The listing builds one solid part. Answer for the finished solid, in the listing's coordinates (mm). A direction names the side the tool comes from. Round coordinates to 2 decimals unless told otherwise and drop trailing zeros. Order: outer loops, then holes, each group sorted by start corner. A loop starts at its lowest first (then second) coordinate and runs counter-clockwise, first axis right, second up. Notation, with made-up numbers: (5, 33.5) -> (25, 33.5) arc R13 cw to (25, 45.5) -> close; hole circle Ø3 at (49, 71). An arc over 180 degrees is marked (long way). Return JSON: item names as keys, results as strings. Group by question number.
(1) Consider line 1 (Y direction, x = 0, z = 2.25); line 2 (Z direction, x = 4.25, y = -2); line 3 (Y direction, x = 0, z = 1.2). Determine where each line is inside the solid, lowest interval first. Write a range as [from, to].
(2) The part is cut by section A-A (z = 2.4). Count the separate pieces of the cut face and the enclosed holes in it, plus the area to 3 significant figures.
(3) The part is cut by section C-C (y = -4). Determine the outline of the cut face in (x, z).
(4) The part is cut by section D-D (y = 5.25). Determine the outline of the cut face in (x, z), plus the area to 3 significant figures.
(5) Each of these flat-tipped pins is pushed along its axis until it touches: pin 1 (4.5 mm diameter, centred on x = 0, y = 0, fed in from -Z); pin 2 (0.9 mm diameter, centred on x = -2, y = 4, fed in from +Z); pin 3 (0.5 mm diameter, centred on x = 1, y = 4, fed in from +Z). Where does it stop, or does it pass through?
(6) Determine the mould class of faces 3 (the face through (0.007, 4.1, 2.745)), 4 (the face through (1.2, -1.2, 1.6)), 5 (the face through (-1, 4, 2.1)), 6 (the face through (-2.894, 2.904, 2.745)) for opening direction X: +X half, -X half, draft (parallel to the pull), parting line (faces both ways), or undercut.
(7) Which of the six approach directions +Z, -Z, +X, -X, +Y, -Y give full straight-line access (tool end or side, diameter ignored) to faces 1 (the face through (4, 1, 2.1)), 2 (the face through (-3, -1, 2.9))?
(8) The part is cut by section B-B (z = 0.95). Determine the outline of the cut face in (x, y), plus the area to 3 significant figures.
from build123d import *

# Parameters (mm, degrees)
PAD008_DEPTH          = 2.6
SKETCH020_R           = 3.625
SKETCH020_R_2         = 2.85
PAD009_DEPTH          = 2.9
SKETCH021_R           = 4.625
SKETCH021_R_2         = 3.625
POCKET011_DEPTH       = 0.5
PAD010_DEPTH          = 0.5
POLARPATTERN006_COUNT = 8
SKETCH023_R           = 2.85
POCKET012_DEPTH       = 1.3
SKETCH024_R           = 1.5
POCKET013_DEPTH       = 5
SKETCH025_R           = 0.75
POCKET014_DEPTH       = 5
POLARPATTERN007_COUNT = 4
SKETCH026_R           = 4.3
PAD011_DEPTH          = 3
POCKET015_DEPTH       = 5
POCKET015_DEPTH_BACK  = 0.5
POLARPATTERN008_COUNT = 25
FILLET001_R           = 1
SKETCH028_R           = 25
SKETCH028_R_2         = 6
POCKET016_DEPTH       = 5


with BuildPart() as part:
    # Sketch019 → Pad008 (new body)
    with BuildSketch(Plane.XY):
        with BuildLine():
            ThreePointArc((3.1440666838, 19.7956884151), (0, 22.4), (-3.1440666838, 19.7956884151))
            Line((-3.1440666838, 19.7956884151), (-5, 10))
            Line((-5, 10), (-5, 5))
            Line((-5, 5), (-10, 5))
            Line((-10, 5), (-19.7956884151, 3.1440666838))
            ThreePointArc((-19.7956884151, 3.1440666838), (-22.4, 0), (-19.7956884151, -3.1440666838))
            Line((-10, -5), (-19.7956884151, -3.1440666838))
            Line((-5, -5), (-10, -5))
            Line((-5, -10), (-5, -5))
            Line((-3.1440666838, -19.7956884151), (-5, -10))
            ThreePointArc((-3.1440666838, -19.7956884151), (0, -22.4), (3.1440666838, -19.7956884151))
            Line((3.1440666838, -19.7956884151), (5, -10))
            Line((5, -10), (5, -5))
            Line((5, -5), (10, -5))
            Line((10, -5), (19.7956884151, -3.1440666838))
            ThreePointArc((19.7956884151, -3.1440666838), (22.4, 0), (19.7956884151, 3.1440666838))
            Line((10, 5), (19.7956884151, 3.1440666838))
            Line((5, 5), (10, 5))
            Line((5, 10), (5, 5))
            Line((3.1440666838, 19.7956884151), (5, 10))
        make_face()
    extrude(amount=PAD008_DEPTH)

    # Sketch020 → Pad009 (join)
    with BuildSketch(Plane.XY):
        Circle(SKETCH020_R)
        Circle(SKETCH020_R_2, mode=Mode.SUBTRACT)
    extrude(amount=PAD009_DEPTH)

    # Sketch021 (on Face5 of Pad009) → Pocket011 (cut)
    with BuildSketch(Plane.XY.offset(2.6)):
        Circle(SKETCH021_R)
        Circle(SKETCH021_R_2, mode=Mode.SUBTRACT)
    extrude(amount=-POCKET011_DEPTH, mode=Mode.SUBTRACT)

    # Sketch022 → Pad010 (join, symmetric)
    with BuildSketch(Plane.XZ):
        Polygon((3.537661, 2.9), (4.625, 2.6), (4.625, 2.1), (3.537661, 2.1), align=None)
    pad010 = extrude(amount=PAD010_DEPTH, both=True)

    # PolarPattern006: Pad010 ×8 about axis
    polarpattern006_axis = Axis((0, 0, 0), (0, 0, 1))
    for i in range(1, POLARPATTERN006_COUNT):
        add(pad010.rotate(polarpattern006_axis, i * 360 / POLARPATTERN006_COUNT))

    # Sketch023 (on Face74 of PolarPattern006) → Pocket012 (cut)
    with BuildSketch(Plane.XY.offset(2.9)):
        Circle(SKETCH023_R)
    extrude(amount=-POCKET012_DEPTH, mode=Mode.SUBTRACT)

    # Sketch024 (on Face66 of Pocket012) → Pocket013 (cut)
    with BuildSketch(Plane.XY.offset(1.6)):
        Circle(SKETCH024_R)
    extrude(amount=-POCKET013_DEPTH, mode=Mode.SUBTRACT)

    # Sketch025 → Pocket014 (cut)
    with BuildSketch(Plane.XY):
        with Locations((8.8, 0)):
            Circle(SKETCH025_R)
        with Locations((12.17411, 0)):
            Circle(SKETCH025_R)
        with Locations((15.54822, 0)):
            Circle(SKETCH025_R)
        with Locations((18.92233, 0)):
            Circle(SKETCH025_R)
    pocket014 = extrude(amount=POCKET014_DEPTH, mode=Mode.SUBTRACT)

    # PolarPattern007: Pocket014 ×4 about axis
    polarpattern007_axis = Axis((0, 0, 0), (0, 0, 1))
    for i in range(1, POLARPATTERN007_COUNT):
        add(pocket014.rotate(polarpattern007_axis, i * 360 / POLARPATTERN007_COUNT), mode=Mode.SUBTRACT)

    # Sketch026 → Pad011 (join)
    with BuildSketch(Plane.XY):
        Circle(SKETCH026_R)
    extrude(amount=-PAD011_DEPTH)

    # Sketch027 → Pocket015 (cut, two sides)
    with BuildSketch(Plane.XY) as pocket015_sk:
        with BuildLine():
            ThreePointArc((2.9950699672, 0.1719182704), (2.9874502188, 0.2741189345), (2.9763441039, 0.3759997007))
            Line((0, 0), (2.9763441039, 0.3759997007))
            Line((0, 0), (2.9763441039, -0.3759997007))
            ThreePointArc((2.9763441039, -0.3759997007), (2.9874502188, -0.2741189345), (2.9950699672, -0.1719182704))
            Line((2.703959, 0), (2.9950699672, -0.1719182704))
            Line((2.9950699672, 0.1719182704), (2.703959, 0))
        make_face()
    pocket015 = extrude(amount=-POCKET015_DEPTH, mode=Mode.SUBTRACT) + extrude(pocket015_sk.sketch, amount=POCKET015_DEPTH_BACK, mode=Mode.SUBTRACT)

    # PolarPattern008: Pocket015 ×25 about axis
    polarpattern008_axis = Axis((0, 0, 0), (0, 0, 1))
    for i in range(1, POLARPATTERN008_COUNT):
        add(pocket015.rotate(polarpattern008_axis, i * 360 / POLARPATTERN008_COUNT), mode=Mode.SUBTRACT)

    # Fillet001
    fillet001_edges = [part.edges().sort_by_distance(p)[0] for p in [
        (-5, -5, 1.3),
        (5, -5, 1.3),
        (5, 5, 1.3),
        (-5, 5, 1.3),
    ]]
    fillet(fillet001_edges, radius=FILLET001_R)

    # Sketch028 → Pocket016 (cut, symmetric)
    with BuildSketch(Plane.XY):
        Circle(SKETCH028_R)
        Circle(SKETCH028_R_2, mode=Mode.SUBTRACT)
    extrude(amount=POCKET016_DEPTH, both=True, mode=Mode.SUBTRACT)


solid = part.part
Answer below:
{
 "1": {"line 1": "y = [-6, -2.85], [2.85, 6]", "line 2": "z = [0, 2.6]", "line 3": "y = [-6, -1.5], [1.5, 6]"},
 "2": {"separate pieces": "1", "enclosed holes": "9", "area": "69.7 mm²"},
 "3": {"outline": "(-4.47, 0) -> (-1.58, 0) -> (-1.58, -3) -> (1.58, -3) -> (1.58, 0) -> (4.47, 0) -> (4.47, 2.6) -> (2.32, 2.6) -> (2.32, 2.1) -> (0.5, 2.1) -> (0.5, 2.77) -> (-0.5, 2.77) -> (-0.5, 2.1) -> (-2.32, 2.1) -> (-2.32, 2.6) -> (-4.47, 2.6) -> close"},
 "4": {"outline": "(-2.9, 0) -> (2.9, 0) -> (2.9, 2.6) -> (-2.9, 2.6) -> close", "area": "15.1 mm²"},
 "5": {"pin 1": "stops at z = 0.5", "pin 2": "stops at z = 2.6", "pin 3": "stops at z = 2.1"},
 "6": {"face 3": "draft", "face 4": "undercut", "face 5": "undercut", "face 6": "-X half"},
 "7": {"face 1": "+Z", "face 2": "+Z, +X, -X, +Y, -Y"},
 "8": {"outline": "circle Ø12 at (0, 0); hole circle Ø3 at (0, 0)", "area": "106 mm²"}
}
